Design review of the part built by this model. Coordinates are the model's own, in mm. A direction names the side the tool comes from. Round coordinates to 2 decimals unless told otherwise and drop trailing zeros. Loops run counter-clockwise (first coordinate to the right, second up) from the corner with the lowest first, then second, coordinate; pieces in that order, holes last. Notation, with made-up numbers: M 87.25,1 L 112.25,1 A14 cw 112.25,8 Z; hole C 50,49.25 d2. An arc over 180 degrees is marked long. Use a Markdown table: item, result.
from build123d import *

# Parameters (mm, degrees)
SKETCH1_W            = 8
SKETCH1_H            = 32
BOSS_EXTRUDE1_DEPTH  = 9.6
SKETCH2_R            = 2.4
BOSS_EXTRUDE2_DEPTH  = 1.6
LPATTERN1_COUNT      = 2
LPATTERN1_PITCH      = 8
LPATTERN1_COUNT_DIR2 = 4
LPATTERN1_PITCH_DIR2 = 8
SHELL1_T             = -1.6


with BuildPart() as part:
    # Sketch1 → Boss-Extrude1 (new body)
    with BuildSketch(Plane(origin=(0, 0, 0), x_dir=(1, 0, 0), z_dir=(0, 1, 0))):
        with Locations((4, 16)):
            Rectangle(SKETCH1_W, SKETCH1_H)
    extrude(amount=BOSS_EXTRUDE1_DEPTH)

    # Sketch2 → Boss-Extrude2 (add)
    with BuildSketch(Plane(origin=(0, 9.6, 0), x_dir=(1, 0, 0), z_dir=(0, 1, 0))):
        with Locations(Location((4, 4, 0), (0, 0, 90))):
            Circle(SKETCH2_R)
    boss_extrude2 = extrude(amount=BOSS_EXTRUDE2_DEPTH)

    # LPattern1: Boss-Extrude2 2 × 4, 4 skipped
    with Locations(*[(i * LPATTERN1_PITCH, 0, -j * LPATTERN1_PITCH_DIR2) for i in range(LPATTERN1_COUNT) for j in range(LPATTERN1_COUNT_DIR2) if (i, j) not in ((0, 0), (1, 0), (1, 1), (1, 2), (1, 3))]):
        add(boss_extrude2)

    # Shell1
    shell1_openings = [part.faces().sort_by_distance(p)[0] for p in [
        (4, 0, -16),
    ]]
    offset(amount=SHELL1_T, openings=shell1_openings, kind=Kind.INTERSECTION)


solid = part.part
1. Take a section at B-B on z = -15.5. Give the boundary of the cut face in (x, y), and give its area (3 significant figures).
Check values:
| item | result |
|---|---|
| outline | M 0,0 L 1.6,0 L 1.6,8 L 6.4,8 L 6.4,0 L 8,0 L 8,9.6 L 0,9.6 Z |
| area | 38.4 mm² |
2. The part is to be moulded in two halves that separate along Z. For faces 4 (the face through (0, 5, -16)), 5 (the face through (4, 9.6, -28)), 6 (the face through (4, 5, 0)), say which applies: pulls with the +Z half, pulls with the -Z half, needs draft (parallel to the pull), parting line crosses it, or undercut.
Check values:
| item | result |
|---|---|
| face 4 | needs draft |
| face 5 | undercut |
| face 6 | pulls with the +Z half |
3. Insertion check: pin 1 (2.5 mm diameter, centred on x = 5, z = -21, fed in from -Y); pin 2 (4 mm diameter, centred on y = 3.5, z = -9, fed in from -X). Each pin has a flat end and moves straight along its axis. Give the tip position at first contact, or say it passes through.
Check values:
| item | result |
|---|---|
| pin 1 | stops at y = 8 |
| pin 2 | stops at x = 0 |
4. Take a section at A-A on y = 1. Give the boundary of the cut face in (x, z).
Check values:
| item | result |
|---|---|
| outline | M 0,-32 L 8,-32 L 8,0 L 0,0 Z; hole M 1.6,-30.4 L 6.4,-30.4 L 6.4,-1.6 L 1.6,-1.6 Z |
5. Take a section at C-C on x = 1.25. Give the boundary of the cut face in (y, z), and give its area (3 significant figures).
Check values:
| item | result |
|---|---|
| outline | M 0,-32 L 9.6,-32 L 9.6,0 L 0,0 Z |
| area | 307 mm² |
6. Take a section at D-D on z = -20. Give the boundary of the cut face in (x, y).
Check values:
| item | result |
|---|---|
| outline | M 0,0 L 1.6,0 L 1.6,8 L 3.2,8 L 3.2,9.6 L 4.8,9.6 L 4.8,8 L 6.4,8 L 6.4,0 L 8,0 L 8,9.6 L 6.4,9.6 L 6.4,11.2 L 1.6,11.2 L 1.6,9.6 L 0,9.6 Z |
7. Machinability: for faces 1 (the face through (4.78, 8.79, -11.83)), 2 (the face through (3.894, 10.389, -25.602)), 3 (the face through (4, 11.2, -12)), which of the approach directions +Z, -Z, +X, -X, +Y, -Y give a long, thin tool a straight path to every point of the face, cutting with its end or side? Answer none if there is none.
Check values:
| item | result |
|---|---|
| face 1 | -Y |
| face 2 | +Y |
| face 3 | +Z, -Z, +X, -X, +Y |
8. Wall thickness on line 1 along X through (y, z) = (0.75, -7); line 2 along X through (y, z) = (8.75, -28); line 3 along Z through (x, y) = (2.25, 5.25): over which ranges is each line inside the solid? List them lowest first. Write a range as from..to.
Check values:
| item | result |
|---|---|
| line 1 | x = 0..1.6, 6.4..8 |
| line 2 | x = 0..3.2, 4.8..8 |
| line 3 | z = -32..-30.4, -1.6..0 |
